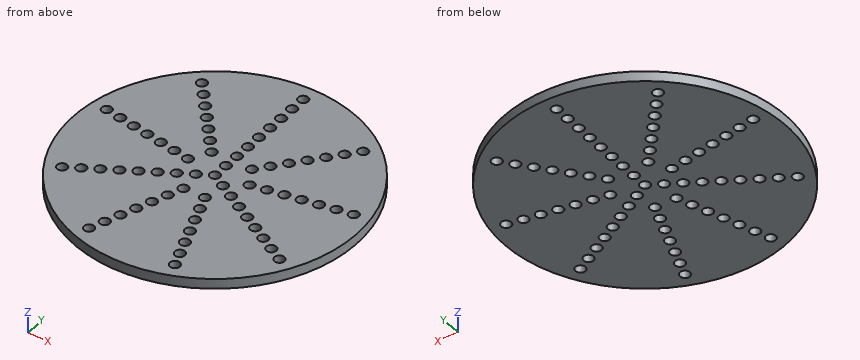
from build123d import *

# Parameters (mm, degrees)
F0_R     = 88.9
F1_DEPTH = 6.35
F2_R     = 3.175
F3_DEPTH = 6.351


with BuildPart() as f1:
    # F0 (on Top) → F1 (new body)
    with BuildSketch(Plane.XY):
        Circle(F0_R)
    extrude(amount=F1_DEPTH)

    # F2 (on face) → F3 (cut, through all)
    with BuildSketch(Plane.XY.offset(6.35)):
        Circle(F2_R)
        with Locations((0, 9.906)):
            Circle(F2_R)
        with Locations((0, 19.812)):
            Circle(F2_R)
        with Locations((0, 29.718)):
            Circle(F2_R)
        with Locations((0, 39.624)):
            Circle(F2_R)
        with Locations((0, 49.53)):
            Circle(F2_R)
        with Locations((0, 59.436)):
            Circle(F2_R)
        with Locations((0, 69.342)):
            Circle(F2_R)
        with Locations((185.832307, 80.557868)):
            Circle(F2_R)
        with Locations((0, 79.248)):
            Circle(F2_R)
        with Locations((-68.630781, -39.624)):
            Circle(F2_R)
        with Locations((-60.051934, -34.671)):
            Circle(F2_R)
        with Locations((-51.473086, -29.718)):
            Circle(F2_R)
        with Locations((-42.894238, -24.765)):
            Circle(F2_R)
        with Locations((-34.315391, -19.812)):
            Circle(F2_R)
        with Locations((-25.736543, -14.859)):
            Circle(F2_R)
        with Locations((-17.157695, -9.906)):
            Circle(F2_R)
        with Locations((-8.578848, -4.953)):
            Circle(F2_R)
        with Locations((68.630781, -39.624)):
            Circle(F2_R)
        with Locations((60.051934, -34.671)):
            Circle(F2_R)
        with Locations((51.473086, -29.718)):
            Circle(F2_R)
        with Locations((42.894238, -24.765)):
            Circle(F2_R)
        with Locations((34.315391, -19.812)):
            Circle(F2_R)
        with Locations((25.736543, -14.859)):
            Circle(F2_R)
        with Locations((17.157695, -9.906)):
            Circle(F2_R)
        with Locations((8.578848, -4.953)):
            Circle(F2_R)
        with Locations((-6.776103, -18.61719)):
            Circle(F2_R)
        with Locations((-10.164155, -27.925785)):
            Circle(F2_R)
        with Locations((-13.552206, -37.23438)):
            Circle(F2_R)
        with Locations((-16.940258, -46.542976)):
            Circle(F2_R)
        with Locations((-20.328309, -55.851571)):
            Circle(F2_R)
        with Locations((-23.716361, -65.160166)):
            Circle(F2_R)
        with Locations((-27.104412, -74.468761)):
            Circle(F2_R)
        with Locations((-12.734908, 15.176873)):
            Circle(F2_R)
        with Locations((-19.102362, 22.765309)):
            Circle(F2_R)
        with Locations((-25.469816, 30.353745)):
            Circle(F2_R)
        with Locations((-31.83727, 37.942181)):
            Circle(F2_R)
        with Locations((-38.204724, 45.530618)):
            Circle(F2_R)
        with Locations((-44.572178, 53.119054)):
            Circle(F2_R)
        with Locations((-50.939632, 60.70749)):
            Circle(F2_R)
        with Locations((19.511011, 3.440318)):
            Circle(F2_R)
        with Locations((29.266517, 5.160477)):
            Circle(F2_R)
        with Locations((39.022022, 6.880635)):
            Circle(F2_R)
        with Locations((48.777528, 8.600794)):
            Circle(F2_R)
        with Locations((58.533034, 10.320953)):
            Circle(F2_R)
        with Locations((68.288539, 12.041112)):
            Circle(F2_R)
        with Locations((78.044045, 13.761271)):
            Circle(F2_R)
        with Locations((-19.511011, 3.440318)):
            Circle(F2_R)
        with Locations((-29.266517, 5.160477)):
            Circle(F2_R)
        with Locations((-39.022022, 6.880635)):
            Circle(F2_R)
        with Locations((-48.777528, 8.600794)):
            Circle(F2_R)
        with Locations((-58.533034, 10.320953)):
            Circle(F2_R)
        with Locations((-68.288539, 12.041112)):
            Circle(F2_R)
        with Locations((-78.044045, 13.761271)):
            Circle(F2_R)
        with Locations((12.734908, 15.176873)):
            Circle(F2_R)
        with Locations((19.102362, 22.765309)):
            Circle(F2_R)
        with Locations((25.469816, 30.353745)):
            Circle(F2_R)
        with Locations((31.83727, 37.942181)):
            Circle(F2_R)
        with Locations((38.204724, 45.530618)):
            Circle(F2_R)
        with Locations((44.572178, 53.119054)):
            Circle(F2_R)
        with Locations((50.939632, 60.70749)):
            Circle(F2_R)
        with Locations((6.776103, -18.61719)):
            Circle(F2_R)
        with Locations((10.164155, -27.925785)):
            Circle(F2_R)
        with Locations((13.552206, -37.23438)):
            Circle(F2_R)
        with Locations((16.940258, -46.542976)):
            Circle(F2_R)
        with Locations((20.328309, -55.851571)):
            Circle(F2_R)
        with Locations((23.716361, -65.160166)):
            Circle(F2_R)
        with Locations((27.104412, -74.468761)):
            Circle(F2_R)
    extrude(amount=-F3_DEPTH, mode=Mode.SUBTRACT)


solid = f1.part
Can you work these out from the model? Positions are in its coordinate system, mm. Round coordinates to 2 decimals unless told otherwise and drop trailing zeros. Use one line per item in the form item = value. Start each with the question number.
Q1. Imagine slicing it at A-A (x = 0). Count the separate pieces of the cut face and the enclosed holes in it, then the cut area to 3 significant figures.
Q2. If I drill on probe 1 along Y at (x, z) = (33, 5); probe 2 along X at (y, z) = (51, 1.5); probe 3 along X at (y, z) = (-33, 3.5), over which ranges is the centre line in solid material (lowest first)? Write a range as [from, to].
Q3. I'm going to push a flat-ended pin straight in: P1, Ø3, axis at y = 54.5, z = 5.5, coming from the -X side. Where does the tip first touch, or does it pass through?
Worked out:
q1.separate_pieces = 10
q1.enclosed_holes = 0
q1.area = 766 mm^2
q2.probe_1 = [-82.55, -22.7], [-16.92, 34.99], [40.9, 82.55]
q2.probe_2 = [-72.82, -46.94], [-42.21, -2.81], [2.81, 42.21], [46.94, 72.82]
q2.probe_3 = [-82.55, -62.75], [-57.35, 57.35], [62.75, 82.55]
q3.P1 = -71.37
